The model under review builds one solid part; all positions refer to its coordinate system, in mm. Face numbers are marked on the shaded views. A direction names the side the tool comes from. Round coordinates to 2 decimals unless told otherwise and drop trailing zeros. Order: outer loops, then holes, each group sorted by start corner. A loop starts at its lowest first (then second) coordinate and runs counter-clockwise, first axis right, second up.
1) Mouldability with a two-part tool opening along X and no side actions: class the marked faces 1, 2 and 3 as pulls with the +X half, pulls with the -X half, needs draft (parallel to the pull), parting line crosses it, or undercut.
2) To check wall thickness, follow L1, parallel to X at y = 2.75, z = 9 (3 decimals); L2, parallel to Z at x = 11, y = 13; L3, parallel to X at y = 14, z = 1.5 (3 decimals). State the ranges of each line that lie inside material, in increasing order.
3) Consider section D-D (z = 15.5). Give the boundary of the cut face in (x, y) (3 decimals).
4) Consider section C-C (y = 14.5). Give the number of separate pieces and of enclosed holes in the cut face, then the cut area to 3 significant figures.
5) Clearance check with flat-ended pins moving along their axes: P1, Ø1.9, axis at x = 6, y = 14, coming from the -Z side; P2, Ø2, axis at x = 9, y = 5, coming from the +Z side; P3, Ø2.5, axis at x = 1, z = 15, coming from the -Y side. State where each tip first meets the part, or that it passes through.
6) Machinability: for the marked faces 4, 5, 6, 7 and 8, which of the approach directions +Z, -Z, +X, -X, +Y, -Y give a long, thin tool a straight path to every point of the face, cutting with its end or side? Answer none if there is none.
7) Consider section B-B (y = 3). Give the boundary of the cut face in (x, z) (1 decimal), then the cut area to 3 significant figures.
8) Consider section A-A (x = 7). Give the boundary of the cut face in (y, z), then the cut area to 3 significant figures.
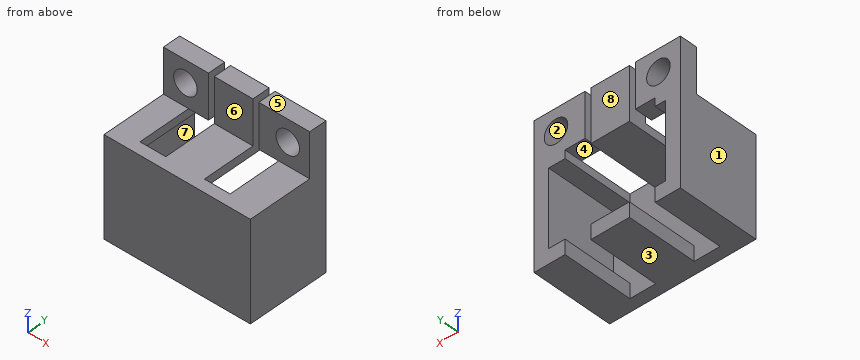
from build123d import *

# Parameters (mm, degrees)
SKETCH1_W              = 31.75
SKETCH1_H              = 21.463
PLATE_DEPTH            = 1.27
SKETCH4_W              = 31.75
SKETCH4_H              = 15.24
BOSS_EXTRUDE1_DEPTH    = 1.778
SKETCH5_W              = 3.175
SKETCH5_H              = 15.24
BOSS_EXTRUDE2_DEPTH    = 19.685
BOSS_EXTRUDE5_REACH    = 36.703
SKETCH9_W              = 3.175
SKETCH9_H              = 15.24
SKETCH11_W             = 5.588
SKETCH11_H             = 15.24
CUT_EXTRUDE1_DEPTH     = 32.388789304
SKETCH13_W             = 31.75
SKETCH13_H             = 3.81
BOSS_EXTRUDE7_DEPTH    = 9.652
F_10_CLEARANCE_HOLE1_D = 5.1054
SKETCH18_W             = 1.27
SKETCH18_H             = 9.652
CUT_EXTRUDE6_DEPTH     = 32.362893636


with BuildPart() as part:
    # Sketch1 → Plate (new, symmetric)
    with BuildSketch(Plane(origin=(0, 0, 0), x_dir=(1, 0, 0), z_dir=(0, 1, 0))):
        Rectangle(SKETCH1_W, SKETCH1_H)
    extrude(amount=PLATE_DEPTH, both=True)

    # Sketch4 → Boss-Extrude1 (add)
    with BuildSketch(Plane.XY.offset(10.7315)):
        with Locations((0, 8.89)):
            Rectangle(SKETCH4_W, SKETCH4_H)
    extrude(amount=-BOSS_EXTRUDE1_DEPTH)

    # Sketch5 → Boss-Extrude2 (add)
    with BuildSketch(Plane(origin=(0, 0, 8.9535), x_dir=(-1, 0, 0), z_dir=(0, 0, -1))):
        with Locations((-14.2875, 8.89)):
            Rectangle(SKETCH5_W, SKETCH5_H)
        with Locations((14.2875, 8.89)):
            Rectangle(SKETCH5_W, SKETCH5_H)
    extrude(amount=BOSS_EXTRUDE2_DEPTH)

    # Sketch9 → Boss-Extrude5 (add, up to next)
    with BuildSketch(Plane.ZY.offset(-12.7), mode=Mode.PRIVATE) as boss_extrude5_sk1:
        with Locations((-9.144, 8.89)):
            Rectangle(SKETCH9_W, SKETCH9_H)
    boss_extrude5_tool1 = extrude(boss_extrude5_sk1.sketch, amount=BOSS_EXTRUDE5_REACH, mode=Mode.PRIVATE) - part.part
    add(boss_extrude5_tool1.solids().sort_by_distance((12.7, 8.89, -9.144))[0])

    # Sketch11 → Cut-Extrude1 (cut, through all)
    with BuildSketch(Plane(origin=(0, 0, -10.7315), x_dir=(-1, 0, 0), z_dir=(0, 0, -1))):
        with Locations((-6.35, 8.89)):
            Rectangle(SKETCH11_W, SKETCH11_H)
        with Locations((7.62, 8.89)):
            Rectangle(SKETCH11_W, SKETCH11_H)
    extrude(amount=-CUT_EXTRUDE1_DEPTH, mode=Mode.SUBTRACT)

    # Sketch13 → Boss-Extrude7 (add)
    with BuildSketch(Plane.XY.offset(10.7315)):
        with Locations((0, 14.605)):
            Rectangle(SKETCH13_W, SKETCH13_H)
    extrude(amount=BOSS_EXTRUDE7_DEPTH)

    # #10 Clearance Hole1 (through all)
    with Locations(Plane(origin=(11.1125, 16.51, 15.621), x_dir=(0, 0, 1), z_dir=(0, 1, 0))):
        with Locations((0, 0), (0, -22.225)):
            Hole(F_10_CLEARANCE_HOLE1_D / 2)

    # Sketch18 → Cut-Extrude6 (cut, through all)
    with BuildSketch(Plane(origin=(0, 16.51, 0), x_dir=(1, 0, 0), z_dir=(0, 1, 0))):
        with Locations((-5.461, -15.5575)):
            Rectangle(SKETCH18_W, SKETCH18_H)
        with Locations((4.191, -15.5575)):
            Rectangle(SKETCH18_W, SKETCH18_H)
    extrude(amount=-CUT_EXTRUDE6_DEPTH, mode=Mode.SUBTRACT)


solid = part.part
Answer below:
1. face 1: pulls with the -X half
1. face 2: undercut
1. face 3: needs draft
2. L1: x = -15.875 to -10.414, -4.826 to 3.556, 9.144 to 15.875
2. L2: z = -10.73 to -7.56, 8.95 to 13.07, 18.17 to 20.38
2. L3: x = -15.875 to -12.7, 12.7 to 15.875
3. outline: (-15.875, 12.7) - (-13.662, 12.7) - (-13.662, 16.51) - (-15.875, 16.51) - close; (-8.563, 12.7) - (-6.096, 12.7) - (-6.096, 16.51) - (-8.563, 16.51) - close; (-4.826, 12.7) - (3.556, 12.7) - (3.556, 16.51) - (-4.826, 16.51) - close; (4.826, 12.7) - (8.563, 12.7) - (8.563, 16.51) - (4.826, 16.51) - close; (13.662, 12.7) - (15.875, 12.7) - (15.875, 16.51) - (13.662, 16.51) - close
4. separate pieces: 4
4. enclosed holes: 2
4. area: 448 mm2
5. P1: stops at z = 10.73
5. P2: stops at z = 10.73
5. P3: stops at y = 12.7
6. face 4: -Z, +Y
6. face 5: +Z, +X, -X, +Y, -Y
6. face 6: +Z, +X, -X, -Y
6. face 7: +Y
6. face 8: +Z, -Z, +X, -X, +Y
7. outline: (-15.9, -10.7) - (-10.4, -10.7) - (-10.4, -7.6) - (-12.7, -7.6) - (-12.7, 9) - (-10.4, 9) - (-10.4, 10.7) - (-15.9, 10.7) - close; (-4.8, -10.7) - (3.6, -10.7) - (3.6, -7.6) - (-4.8, -7.6) - close; (-4.8, 9) - (3.6, 9) - (3.6, 10.7) - (-4.8, 10.7) - close; (9.1, -10.7) - (15.9, -10.7) - (15.9, 10.7) - (9.1, 10.7) - (9.1, 9) - (12.7, 9) - (12.7, -7.6) - (9.1, -7.6) - close
7. area: 207 mm2
8. outline: (-1.27, -10.73) - (1.27, -10.73) - (1.27, 10.73) - (-1.27, 10.73) - close; (12.7, 10.73) - (16.51, 10.73) - (16.51, 20.38) - (12.7, 20.38) - close
8. area: 91.3 mm2
